```python
from build123d import *

# Parameters (mm, degrees)
Y_KSEKLIK_EKSTR_ZYON1_DEPTH      = 1
Y_KSEKLIK_EKSTR_ZYON1_DEPTH_BACK = 12
IZIM3_W                          = 3
IZIM3_H                          = 10
RADYUS1_R                        = 3
IZIM4_R                          = 1.7
KES_EKSTR_ZYON1_DEPTH            = 31


with BuildPart() as part:
    # Loft1: read off the stored shape, not the designer's step
    # Loft1: loft between two sections, ruled curve by curve
    loft1_from = [
        Edge.make_bspline([(-13, 0, 0), (-13.209224756, 0, 0), (-13.54255809, 0, 0), (-13.875891423, 0, 0), (-14.101661333, 0, 0), (-14.434994666, 0, 0), (-14.768328, 0, 0), (-15, 0, 0)], [0, 0, 0, 0, 0.313837134, 0.5, 0.5, 0.652492, 1, 1, 1, 1], 3),
        Edge.make_bspline([(-15, 0, 0), (-15, -0.406070992, 0), (-14.983401695, -0.812808246, 0), (-14.917335296, -1.623604412, 0), (-14.867867201, -2.027663325, 0), (-14.80212762, -2.428377634, 0)], [0, 0, 0, 0, 0.5, 0.5, 1, 1, 1, 1], 3),
        Edge.make_bspline([(13, 0, 0), (13, -0.541666667, 0), (12.966403007, -1.117524212, 0), (12.803508497, -2.333803221, 0), (12.674133333, -2.9744, 0), (12.285866667, -4.3056, 0), (12.026764297, -4.996380928, 0), (11.344022219, -6.396877499, 0), (10.92, -7.106666667, 0), (9.88, -8.493333333, 0), (9.263526615, -9.170013136, 0), (7.832363796, -10.41902796, 0), (7.017301038, -10.99077278, 0), (5.21799308, -11.950403691, 0), (4.233846154, -12.337435897, 0), (2.166153846, -12.862564103, 0), (1.083333333, -13, 0), (-1.083333333, -13, 0), (-2.166153846, -12.862564103, 0), (-4.233846154, -12.337435897, 0), (-5.21799308, -11.950403691, 0), (-7.017301038, -10.99077278, 0), (-7.832363796, -10.41902796, 0), (-9.263526615, -9.170013136, 0), (-9.88, -8.493333333, 0), (-10.92, -7.106666667, 0), (-11.344022219, -6.396877499, 0), (-12.026764297, -4.996380928, 0), (-12.285866667, -4.3056, 0), (-12.674133333, -2.9744, 0), (-12.803508497, -2.333803221, 0), (-12.966403007, -1.117524212, 0), (-13, -0.541666667, 0), (-13, 0, 0)], [0, 0, 0, 0, 0.0625, 0.0625, 0.125, 0.125, 0.1875, 0.1875, 0.25, 0.25, 0.3125, 0.3125, 0.375, 0.375, 0.4375, 0.4375, 0.5, 0.5, 0.5625, 0.5625, 0.625, 0.625, 0.6875, 0.6875, 0.75, 0.75, 0.8125, 0.8125, 0.875, 0.875, 0.9375, 0.9375, 1, 1, 1, 1], 3),
        Edge.make_bspline([(-14.80212762, -2.428377634, 0), (-14.681938937, -3.16098536, 0), (-14.504127476, -3.902792163, 0), (-14.02427913, -5.377833707, 0), (-13.722166884, -6.11096882, 0), (-12.993207628, -7.537795397, 0), (-12.566336555, -8.231351462, 0), (-11.597614897, -9.547946899, 0), (-11.055808561, -10.170847244, 0), (-9.876980677, -11.319111684, 0), (-9.240065749, -11.844371923, 0), (-7.898482942, -12.778181737, 0), (-7.193955206, -13.18669073, 0), (-5.748476154, -13.877925848, 0), (-5.007659558, -14.160679583, 0), (-3.520524561, -14.601623448, 0), (-2.774303774, -14.75989153, 0), (-2.038792236, -14.860798304, 0)], [0, 0, 0, 0, 0.125, 0.125, 0.25, 0.25, 0.375, 0.375, 0.5, 0.5, 0.625, 0.625, 0.75, 0.75, 0.875, 0.875, 1, 1, 1, 1], 3),
        Edge.make_bspline([(-2.038792236, -14.860798304, 0), (0.134662487, -15.158980307, 0), (2.321229161, -14.980811498, 0), (4.417739539, -14.33469837, 0)], [0, 0, 0, 0, 1, 1, 1, 1], 3, [1, 0.984272414, 0.984272414, 1]),
        Edge.make_bspline([(4.417739539, -14.33469837, 0), (5.127212599, -14.116049389, 0), (5.83796731, -13.839062041, 0), (7.234099562, -13.16317986, 0), (7.919368159, -12.764223905, 0), (9.233873859, -11.848095943, 0), (9.86297355, -11.3309185, 0), (11.035682686, -10.192235719, 0), (11.579160408, -9.570793115, 0), (12.556543149, -8.246833378, 0), (12.990359766, -7.544435992, 0), (13.733156479, -6.088380279, 0), (14.042115417, -5.334866309, 0), (14.53046703, -3.808849147, 0), (14.70990537, -3.036475671, 0), (14.944626607, -1.503208594, 0), (15, -0.742401104, 0), (15, 0, 0)], [0, 0, 0, 0, 0.125, 0.125, 0.25, 0.25, 0.375, 0.375, 0.5, 0.5, 0.625, 0.625, 0.75, 0.75, 0.875, 0.875, 1, 1, 1, 1], 3),
        Edge.make_bspline([(14.691051451, 0, 0), (14.409209542, 0, 0), (14.127367634, 0, 0), (13.563683817, 0, 0), (13.281841908, 0, 0), (13, 0, 0)], [0, 0, 0, 0, 0.5, 0.5, 1, 1, 1, 1], 3),
        Edge.make_line((14.691051451, 0, 0), (15, 0, 0)),
    ]
    loft1_to = [
        Edge.make_bspline([(-12.275322713, -8.62069906, 50), (-13.30009489, -7.9994122, 50), (-14.838773196, -6.851542234, 50), (-16.153887151, -5.461933248, 50), (-16.982212381, -4.468717424, 50), (-18.129692881, -2.939391702, 50), (-19.010068808, -1.232828152, 50), (-19.501011098, 0, 50)], [0, 0, 0, 0, 0.313837134, 0.5, 0.5, 0.652492, 1, 1, 1, 1], 3),
        Edge.make_bspline([(-19.501011098, 0, 50), (-20.001011098, 0, 50), (-20.501011098, 0, 50), (-21.501011098, 0, 50), (-22.001011098, 0, 50), (-22.501011098, 0, 50)], [0, 0, 0, 0, 0.5, 0.5, 1, 1, 1, 1], 3),
        Edge.make_bspline([(7.170134264, -10.843854234, 50), (6.75061217, -10.971235531, 50), (6.331990602, -11.087760763, 50), (5.496548516, -11.2990991, 50), (5.079727998, -11.393912204, 50), (4.247888014, -11.561826283, 50), (3.832868547, -11.634927259, 50), (3.004630665, -11.75941708, 50), (2.591412249, -11.810805927, 50), (1.766776468, -11.891871491, 50), (1.355359103, -11.921548209, 50), (0.534325424, -11.959189516, 50), (0.12470911, -11.967154105, 50), (-0.692722467, -11.961371154, 50), (-1.100537731, -11.947623615, 50), (-1.914367207, -11.898416407, 50), (-2.320381419, -11.862956738, 50), (-3.130608793, -11.770325273, 50), (-3.534821955, -11.713153476, 50), (-4.341447227, -11.577097753, 50), (-4.743859338, -11.498213827, 50), (-5.546882508, -11.318733846, 50), (-5.947493568, -11.218137792, 50), (-6.746914637, -10.995233554, 50), (-7.145724646, -10.87292537, 50), (-7.941543614, -10.606596875, 50), (-8.338552572, -10.462576563, 50), (-9.130769437, -10.15282381, 50), (-9.525977345, -9.987091369, 50), (-10.314592108, -9.633914359, 50), (-10.707998965, -9.446469789, 50), (-11.493011627, -9.049868521, 50), (-11.884617433, -8.840711823, 50), (-12.275322713, -8.62069906, 50)], [0, 0, 0, 0, 0.0625, 0.0625, 0.125, 0.125, 0.1875, 0.1875, 0.25, 0.25, 0.3125, 0.3125, 0.375, 0.375, 0.4375, 0.4375, 0.5, 0.5, 0.5625, 0.5625, 0.625, 0.625, 0.6875, 0.6875, 0.75, 0.75, 0.8125, 0.8125, 0.875, 0.875, 0.9375, 0.9375, 1, 1, 1, 1], 3),
        Edge.make_bspline([(-22.501011098, 0, 50), (-22.201916292, -1.005484405, 50), (-21.843929165, -1.960557007, 50), (-21.010170267, -3.769878608, 50), (-20.534398496, -4.624127606, 50), (-19.465070311, -6.231801999, 50), (-18.871513898, -6.985227394, 50), (-17.566616427, -8.391254578, 50), (-16.85527537, -9.043856368, 50), (-15.314808613, -10.248236345, 50), (-14.485682914, -10.800014531, 50), (-12.709646871, -11.802747299, 50), (-11.762736528, -12.253701882, 50), (-9.751131199, -13.054787442, 50), (-8.686436212, -13.40491842, 50), (-6.439261597, -14.004356772, 50), (-5.256781968, -14.253664146, 50), (-4.015410017, -14.452559718, 50)], [0, 0, 0, 0, 0.125, 0.125, 0.25, 0.25, 0.375, 0.375, 0.5, 0.5, 0.625, 0.625, 0.75, 0.75, 0.875, 0.875, 1, 1, 1, 1], 3),
        Edge.make_bspline([(-4.015410017, -14.452559718, 50), (-1.371847999, -15.187030678, 50), (1.371847999, -15.187030678, 50), (4.015410017, -14.452559718, 50)], [0, 0, 0, 0, 1, 1, 1, 1], 3, [1, 0.975669321, 0.975669321, 1]),
        Edge.make_bspline([(4.015410017, -14.452559718, 50), (5.256781968, -14.253664146, 50), (6.439261597, -14.004356772, 50), (8.686436212, -13.40491842, 50), (9.751131199, -13.054787442, 50), (11.762736528, -12.253701882, 50), (12.709646871, -11.802747299, 50), (14.485682914, -10.800014531, 50), (15.314808613, -10.248236345, 50), (16.85527537, -9.043856368, 50), (17.566616427, -8.391254578, 50), (18.871513898, -6.985227394, 50), (19.465070311, -6.231801999, 50), (20.534398496, -4.624127606, 50), (21.010170267, -3.769878608, 50), (21.843929165, -1.960557007, 50), (22.201916292, -1.005484405, 50), (22.501011098, 0, 50)], [0, 0, 0, 0, 0.125, 0.125, 0.25, 0.25, 0.375, 0.375, 0.5, 0.5, 0.625, 0.625, 0.75, 0.75, 0.875, 0.875, 1, 1, 1, 1], 3),
        Edge.make_bspline([(19.501011098, 0, 50), (18.422591042, -2.708071054, 50), (16.855807944, -4.965761101, 50), (12.745515666, -8.580379179, 50), (10.202006485, -9.93730721, 50), (7.170134264, -10.843854234, 50)], [0, 0, 0, 0, 0.5, 0.5, 1, 1, 1, 1], 3),
        Edge.make_line((19.501011098, 0, 50), (22.501011098, 0, 50)),
    ]
    loft1 = Solid(Shell([*[Face.make_surface_from_curves(loft1_from[k], loft1_to[k]) for k in range(8)], Face(Wire(loft1_from)), Face(Wire(loft1_to))]))
    add(loft1)

    # Çizim3 → Yükseklik-Ekstrüzyon1 (add, two sides: drawn at the far end of the back side and taken through both)
    with BuildSketch(Plane(origin=(0, -15, 0), x_dir=(1, 0, 0), z_dir=(0, 1, 0)).offset(-Y_KSEKLIK_EKSTR_ZYON1_DEPTH_BACK)):
        with Locations((-4.5, -18)):
            Rectangle(IZIM3_W, IZIM3_H)
        with Locations((4.5, -18)):
            Rectangle(IZIM3_W, IZIM3_H)
    extrude(amount=Y_KSEKLIK_EKSTR_ZYON1_DEPTH + Y_KSEKLIK_EKSTR_ZYON1_DEPTH_BACK)

    # Radyus1
    radyus1_edges = [part.edges().sort_by_distance(p)[0] for p in [
        (4.5, -27, 23),
        (4.5, -27, 13),
        (-4.5, -27, 13),
        (-4.5, -27, 23),
    ]]
    fillet(radyus1_edges, radius=RADYUS1_R)

    # Çizim4 → Kes-Ekstrüzyon1 (cut)
    with BuildSketch(Plane.ZY.offset(6)):
        with Locations((18, -23)):
            Circle(IZIM4_R)
    extrude(amount=-KES_EKSTR_ZYON1_DEPTH, mode=Mode.SUBTRACT)


solid = part.part
```
Design review of the part built by this model. Coordinates are the model's own, in mm. A direction names the side the tool comes from. Coordinates: 2 decimals unless noted, no trailing zeros. Order: outer loops, then holes, each group sorted by start corner. A loop starts at its lowest first (then second) coordinate and runs counter-clockwise, first axis right, second up.
1) For faces 1 (the flat face through (6, -21, 18)), 2 (the flat face through (-6, -21, 18)), 3 (the flat face through (4, -27, 18)), 4 (the flat face through (-3, -21, 18)), list the 3-axis set-ups (+Z, -Z, +X, -X, +Y, -Y) from which the entire face can be reached by the end or side of a thin tool; tool diameter is ignored.
2) Wall thickness on line 1 along X through (y, z) = (-4.25, 18); line 2 along X through (y, z) = (-20, 16); line 3 along Y through (x, z) = (17, 47.5): over which ranges is each line inside the solid? List them lowest first.
3) Take a section at A-A, the plane y = -23. Give the boundary of the cut face in (x, z).
4) Mouldability with a two-part tool opening along Y and no side actions: class faces 5 (the flat face through (-5, -27, 18)), 6 (the cylindrical face through (4.48, -23.65, 19.57)), 7 (the cylindrical face through (-4.52, -23.65, 19.57)), 8 (the flat face through (-5, -19, 23)) as +Y half, -Y half, draft (parallel to the pull), parting line (faces both ways), or undercut.
5) Take a section at B-B, the plane z = 18. State how many separate pieces and enclosed holes the cut face has, and give its area (3 significant figures).
6) Clearance check with flat-ended pins moving along their axes: pin 1 (3.5 mm diameter, centred on x = 4.5, y = -17, fed in from -Z); pin 2 (1 mm diameter, centred on x = 14.5, z = 32, fed in from +Y); pin 3 (6 mm diameter, centred on y = -10.5, z = 14.5, fed in from +X). State where each tip first meets the part, or that it passes through.
Returned:
1. face 1: +Z, -Z, +X, -Y
1. face 2: +Z, -Z, -X, -Y
1. face 3: +Z, -Z, +X, -X, -Y
1. face 4: +Z, -Z, -Y
2. line 1: x = -16.75 to -12.32, 10.76 to 16.61
2. line 2: x = -6 to -3, 3 to 6
2. line 3: y = -8.64 to -4.03
3. outline: (-6, 13) - (-3, 13) - (-3, 16.3) - (-6, 16.3) - close; (-6, 19.7) - (-3, 19.7) - (-3, 23) - (-6, 23) - close; (3, 13) - (6, 13) - (6, 16.3) - (3, 16.3) - close; (3, 19.7) - (6, 19.7) - (6, 23) - (3, 23) - close
4. face 5: -Y half
4. face 6: undercut
4. face 7: undercut
4. face 8: draft
5. separate pieces: 3
5. enclosed holes: 0
5. area: 201 mm2
6. pin 1: stops at z = 13
6. pin 2: stops at y = -3.86
6. pin 3: stops at x = 14.51
